Verification items for the finished model (mm, model axes). Face numbers are marked on the shaded views. Give positions to 0.01 mm unless a question says otherwise; leave off trailing zeros. Loops run counter-clockwise (first coordinate to the right, second up) from the corner with the lowest first, then second, coordinate; pieces in that order, holes last. Notation, with made-up numbers: (43.5, 75) - (60.5, 75) arc R12 ccw to (60.5, 94) - close; hole circle Ø7 at (-12.75, 49). An arc over 180 degrees is marked (long way). One line per question, with ' | ' between items. Start each with the question number.
1. Section check A-A, the plane y = 8. Enter the section's corners in (x, z).
2. Section check C-C, the plane x = -43. Enter the section's corners in (y, z).
3. Depth check by flat-ended pin: pin 1 Ø3 at (x, z) = (-68.98, 110.6) entering from -Y; pin 2 Ø8.5 at (x, z) = (64, -45) entering from +Y; pin 3 Ø0.8 at (x, y) = (-26.5, 2) entering from -Z; pin 4 Ø4 at (x, y) = (5.5, 2.5) entering from +Z. Enter the tip coordinate at first touch or a pass-through.
4. Section check D-D, the plane z = -15. Enter the section's corners in (x, y), then the cut area to 3 significant figures.
5. Thickness scan on line 1 along X through (y, z) = (0.5, 29); line 2 along Z through (x, y) = (72, 6.75); line 3 along Z through (x, y) = (-73, 9.25). Record the ranges inside material, lowest first. Write a range as from..to.
6. Section check B-B, the plane z = 97. Enter the section's corners in (x, y), then the cut area to 3 significant figures.
7. Mould release check, pull along Z, two halves, no side actions. Record for the marked faces 1 and 2: +Z half, -Z half, draft (parallel to the pull), parting line (faces both ways), or undercut.
from build123d import *
from build123d.topology import SkipClean

# Parameters (mm, degrees)
BOSS_EXTRUDE1_DEPTH    = 5
M3_TAPPED_HOLE1_D      = 2.5
SKETCH2_R              = 13.95
BOSS_EXTRUDE4_DEPTH    = 5
CUT_EXTRUDE1_START     = -5
CUT_EXTRUDE1_OUTLINE_W = 2.807246308
CUT_EXTRUDE1_OUTLINE_H = 24.121523831
CUT_EXTRUDE1_DEPTH     = 5


# Read off the part's stored shape, not the designer's step: Cut-Extrude1
with BuildPart() as part:
    # Sketch1 → Boss-Extrude1 (new body)
    with BuildSketch(Plane(origin=(0, 0, 0), x_dir=(1, 0, 0), z_dir=(0, 1, 0))):
        with BuildLine():
            Line((-15, 7.390657387), (15, 7.390657387))
            Line((15, 7.390657387), (58.070303134, 56.072779239))
            ThreePointArc((58.070303134, 56.072779239), (79.243939669, 57.367814327), (80.538974758, 36.194177792))
            Line((80.538974758, 36.194177792), (37.468671624, -12.487944059))
            Line((37.468671624, -12.487944059), (37.468671624, -42.487944059))
            Line((37.468671624, -42.487944059), (80.538974758, -91.17006591))
            ThreePointArc((80.538974758, -91.17006591), (79.243939669, -112.343702445), (58.070303134, -111.048667357))
            Line((58.070303134, -111.048667357), (15, -62.366545506))
            Line((15, -62.366545506), (-15, -62.366545506))
            Line((-15, -62.366545506), (-58.070303134, -111.048667357))
            ThreePointArc((-58.070303134, -111.048667357), (-79.243939669, -112.343702445), (-80.538974758, -91.17006591))
            Line((-80.538974758, -91.17006591), (-37.468671624, -42.487944059))
            Line((-37.468671624, -42.487944059), (-37.468671624, -12.487944059))
            Line((-37.468671624, -12.487944059), (-80.538974758, 36.194177792))
            ThreePointArc((-80.538974758, 36.194177792), (-79.243939669, 57.367814327), (-58.070303134, 56.072779239))
            Line((-58.070303134, 56.072779239), (-15, 7.390657387))
        make_face()
    extrude(amount=BOSS_EXTRUDE1_DEPTH)

    # M3 Tapped Hole1 (through all)
    with Locations(Plane(origin=(-77.299965137, 5, -46.406899623), x_dir=(0, 0, 1), z_dir=(0, 1, 0))):
        with Locations((0, 0), (0.273421108, 7.995326191), (-9.221028744, 8.320013756), (0.546842215, 15.990652382), (9.767870959, 7.670638626), (138.021816405, 7.670638626), (147.789687364, 0), (157.010716108, 8.320013756), (147.242845149, 15.990652382), (138.021816405, 146.929291648), (147.242845149, 138.609277892), (147.516266257, 146.604604083), (157.010716108, 146.279916518), (147.789687364, 154.599930274), (0.546842215, 138.609277892), (0.273421108, 146.604604083), (-9.221028744, 146.279916518), (9.767870959, 146.929291648), (0, 154.599930274)):
            Hole(M3_TAPPED_HOLE1_D / 2)

    # Sketch2 → Boss-Extrude4 (add)
    # profile 1 of 4: a face of its own
    with BuildSketch(Plane(origin=(0, 5, 0), x_dir=(1, 0, 0), z_dir=(0, 1, 0))):
        with BuildLine():
            ThreePointArc((-58.070303134, 56.072779239), (-59.365338223, 34.899142704), (-80.538974758, 36.194177792))
            ThreePointArc((-80.538974758, 36.194177792), (-79.243939669, 57.367814327), (-58.070303134, 56.072779239))
        make_face()
        with Locations(Location((-69.304638946, 46.133478515, 0), (0, 0, 270))):
            Circle(SKETCH2_R, mode=Mode.SUBTRACT)
    # profile 2 of 4: a face of its own
    with BuildSketch(Plane(origin=(0, 5, 0), x_dir=(1, 0, 0), z_dir=(0, 1, 0))):
        with BuildLine():
            ThreePointArc((-58.070303134, -111.048667357), (-59.365338223, -89.875030822), (-80.538974758, -91.17006591))
            ThreePointArc((-80.538974758, -91.17006591), (-79.243939669, -112.343702445), (-58.070303134, -111.048667357))
        make_face()
        with Locations(Location((-69.304638946, -101.109366634, 0), (0, 0, 270))):
            Circle(SKETCH2_R, mode=Mode.SUBTRACT)
    # profile 3 of 4: a face of its own
    with BuildSketch(Plane(origin=(0, 5, 0), x_dir=(1, 0, 0), z_dir=(0, 1, 0))):
        with BuildLine():
            ThreePointArc((58.070303134, -111.048667357), (59.365338223, -89.875030822), (80.538974758, -91.17006591))
            ThreePointArc((80.538974758, -91.17006591), (79.243939669, -112.343702445), (58.070303134, -111.048667357))
        make_face()
        with Locations(Location((69.304638946, -101.109366634, 0), (0, 0, 270))):
            Circle(SKETCH2_R, mode=Mode.SUBTRACT)
    # profile 4 of 4: a face of its own
    with BuildSketch(Plane(origin=(0, 5, 0), x_dir=(1, 0, 0), z_dir=(0, 1, 0))):
        with BuildLine():
            ThreePointArc((58.070303134, 56.072779239), (59.365338223, 34.899142704), (80.538974758, 36.194177792))
            ThreePointArc((80.538974758, 36.194177792), (79.243939669, 57.367814327), (58.070303134, 56.072779239))
        make_face()
        with Locations(Location((69.304638946, 46.133478515, 0), (0, 0, 270))):
            Circle(SKETCH2_R, mode=Mode.SUBTRACT)
    extrude(amount=BOSS_EXTRUDE4_DEPTH)

    # Cut-Extrude1 outline → Cut-Extrude1 (cut)
    with SkipClean():  # the faces are left unmerged after this step: merging them gives an invalid solid
        with BuildSketch(Plane(origin=(0, 5, 0), x_dir=(1, 0, 0), z_dir=(0, 1, 0)).offset(CUT_EXTRUDE1_START)):
            with BuildLine():
                ThreePointArc((-50.155470131, 9.911625133), (-45.783130536, 19.029963413), (-36.371791915, 22.729713658))
                ThreePointArc((-36.371791915, 22.729713658), (-35.321791915, 23.779713658), (-36.371791915, 24.829713658))
                ThreePointArc((-36.371791915, 24.829713658), (-47.213213279, 20.567774633), (-52.249943738, 10.063875941))
                ThreePointArc((-52.249943738, 10.063875941), (-51.278832338, 8.940513734), (-50.155470131, 9.911625133))
            make_face()
            with Locations((26.180408459, -29.623395638)):
                Rectangle(CUT_EXTRUDE1_OUTLINE_W, CUT_EXTRUDE1_OUTLINE_H)
            with Locations((-26.533438878, -29.623395638)):
                Rectangle(CUT_EXTRUDE1_OUTLINE_W, CUT_EXTRUDE1_OUTLINE_H)
            with BuildLine():
                ThreePointArc((52.249943738, 10.063875941), (47.213213279, 20.567774633), (36.371791915, 24.829713658))
                ThreePointArc((36.371791915, 24.829713658), (35.321791915, 23.779713658), (36.371791915, 22.729713658))
                ThreePointArc((36.371791915, 22.729713658), (45.783130536, 19.029963413), (50.155470131, 9.911625133))
                ThreePointArc((50.155470131, 9.911625133), (51.278832338, 8.940513734), (52.249943738, 10.063875941))
            make_face()
            with BuildLine():
                ThreePointArc((50.155470131, -64.964128793), (45.783130536, -74.082467073), (36.371791915, -77.782217317))
                ThreePointArc((36.371791915, -77.782217317), (35.321791915, -78.832217317), (36.371791915, -79.882217317))
                ThreePointArc((36.371791915, -79.882217317), (47.213213279, -75.620278293), (52.249943738, -65.116379601))
                ThreePointArc((52.249943738, -65.116379601), (51.278832338, -63.993017394), (50.155470131, -64.964128793))
            make_face()
            with BuildLine():
                ThreePointArc((-52.249943738, -65.116379601), (-47.213213279, -75.620278293), (-36.371791915, -79.882217317))
                ThreePointArc((-36.371791915, -79.882217317), (-35.321791915, -78.832217317), (-36.371791915, -77.782217317))
                ThreePointArc((-36.371791915, -77.782217317), (-45.783130536, -74.082467073), (-50.155470131, -64.964128793))
                ThreePointArc((-50.155470131, -64.964128793), (-51.278832338, -63.993017394), (-52.249943738, -65.116379601))
            make_face()
        extrude(amount=CUT_EXTRUDE1_DEPTH, mode=Mode.SUBTRACT)


solid = part.part
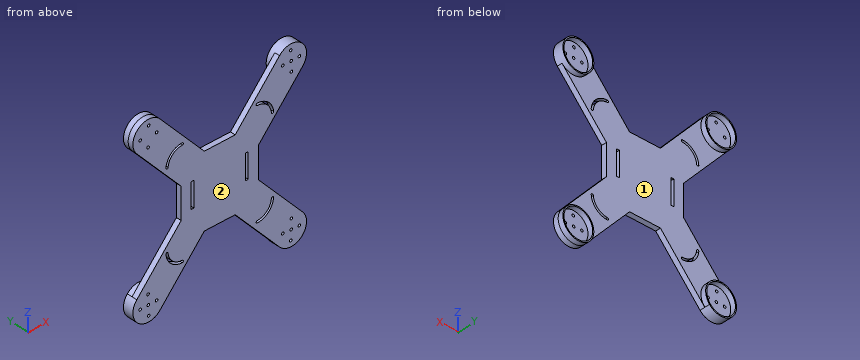
Results list:
1) outline: circle Ø30 at (-69.3, -46.13); circle Ø30 at (-69.3, 101.11); circle Ø30 at (69.3, -46.13); circle Ø30 at (69.3, 101.11); hole circle Ø27.9 at (-69.3, -46.13); hole circle Ø27.9 at (-69.3, 101.11); hole circle Ø27.9 at (69.3, -46.13); hole circle Ø27.9 at (69.3, 101.11)
2) outline: (0, -39.04) - (5, -39.04) - (5, -23.38) - (0, -23.38) - close; (0, -21.04) - (5, -21.04) - (5, 6.24) - (0, 6.24) - close; (0, 48.74) - (5, 48.74) - (5, 76.09) - (0, 76.09) - close; (0, 78.44) - (5, 78.44) - (5, 94.01) - (0, 94.01) - close
3) pin 1: y = 0 | pin 2: y = 5 | pin 3: z = -20.84 | pin 4: z = 62.37
4) outline: (-61.79, 0) - (-51.08, 0) - (-51.08, 5) - (-61.79, 5) - close; (-48.78, 0) - (-21.73, 0) - (-21.73, 5) - (-48.78, 5) - close; (21.73, 0) - (48.78, 0) - (48.78, 5) - (21.73, 5) - close; (51.08, 0) - (61.79, 0) - (61.79, 5) - (51.08, 5) - close | area: 378 mm²
5) line 1: -37.47..-27.94, -25.13..24.78, 27.58..37.47 | line 2: -60.89..-59.82, -32.45..-31.38, 86.35..87.42, 114.8..115.87 | line 3: -60.67..-59.59, -32.68..-31.6, 86.57..87.66, 114.56..115.65
6) outline: (-83.73, 0) - (-45.64, 0) - (-45.64, 5) - (-54.88, 5) - (-54.88, 10) - (-55.97, 10) - (-55.97, 5) - (-82.64, 5) - (-82.64, 10) - (-83.73, 10) - close; (45.64, 0) - (83.73, 0) - (83.73, 10) - (82.64, 10) - (82.64, 5) - (55.97, 5) - (55.97, 10) - (54.88, 10) - (54.88, 5) - (45.64, 5) - close | area: 403 mm²
7) face 1: undercut | face 2: draft
